Build history of the part. All positions in model axes, mm. Round coordinates to 2 decimals unless told otherwise and drop trailing zeros. Loops run counter-clockwise (first coordinate to the right, second up) from the corner with the lowest first, then second, coordinate; pieces in that order, holes last. Notation, with made-up numbers: (-27.5, -6) - (26.5, -6) arc R21 ccw to (26.5, 28) - close; hole circle Ø8 at (60.5, 83). An arc over 180 degrees is marked (long way). Use a Markdown table: item, result.
from build123d import *

# Parameters (mm, degrees)
F0_W     = 1
F0_H     = 5
F1_DEPTH = 2
F2_DEPTH = 2


# Not quite as in the source:
# - a feature names something its author has since deleted; it is built from what else it names


with BuildPart() as f1:
    # F0 (on Front) → F1 (new body)
    with BuildSketch(Plane.XZ):
        Polygon((-11.0105917081, 20.8667229116), (-10.0105917081, 20.8667229116), (-10.0105917081, 15.8667229116), (-10.0105917081, -14.7727085277), (-10.0105917081, -21.2332770884), (9.9894082919, -21.2332770884), (9.9894082919, -23.2332770884), (37.9894082919, -23.2332770884), (65.9894082919, -23.2332770884), (65.9894082919, -21.2332770884), (85.9894082919, -21.2332770884), (85.9894082919, -14.7727085277), (85.9894082919, 15.8667229116), (98.9894082919, 15.8667229116), (103.9894082919, 15.8667229116), (105.0934082919, 15.8667229116), (105.0934082919, 42.8667229116), (103.9894082919, 42.8667229116), (98.9894082919, 42.8667229116), (93.9894082919, 42.8667229116), (37.9894082919, 42.8667229116), (-10.0105917081, 42.8667229116), (-11.0105917081, 42.8667229116), align=None)
        with BuildLine():
            ThreePointArc((46.4894082919, 29.3667229116), (45.4894082919, 28.3667229116), (44.4894082919, 29.3667229116))
            ThreePointArc((44.4894082919, 29.3667229116), (45.4894082919, 30.3667229116), (46.4894082919, 29.3667229116))
        make_face(mode=Mode.SUBTRACT)
        with BuildLine():
            ThreePointArc((93.9894082919, 28.3667229116), (93.2823015107, 30.0738296928), (94.9894082919, 29.3667229116))
            ThreePointArc((94.9894082919, 29.3667229116), (94.6965150731, 28.6596161304), (93.9894082919, 28.3667229116))
        make_face(mode=Mode.SUBTRACT)
        with Locations((-10.5105917081, 18.3667229116)):
            Rectangle(F0_W, F0_H)
    extrude(amount=F1_DEPTH)

    # F0 (on Front) → F2 (join)
    with BuildSketch(Plane.XZ):
        Polygon((-11.0105917081, 20.8667229116), (-10.0105917081, 20.8667229116), (-10.0105917081, 15.8667229116), (-10.0105917081, -14.7727085277), (-10.0105917081, -21.2332770884), (9.9894082919, -21.2332770884), (9.9894082919, -23.2332770884), (37.9894082919, -23.2332770884), (65.9894082919, -23.2332770884), (65.9894082919, -21.2332770884), (85.9894082919, -21.2332770884), (85.9894082919, -14.7727085277), (85.9894082919, 15.8667229116), (98.9894082919, 15.8667229116), (103.9894082919, 15.8667229116), (105.0934082919, 15.8667229116), (105.0934082919, 42.8667229116), (103.9894082919, 42.8667229116), (98.9894082919, 42.8667229116), (93.9894082919, 42.8667229116), (37.9894082919, 42.8667229116), (-10.0105917081, 42.8667229116), (-11.0105917081, 42.8667229116), align=None)
        with BuildLine():
            ThreePointArc((46.4894082919, 29.3667229116), (45.4894082919, 28.3667229116), (44.4894082919, 29.3667229116))
            ThreePointArc((44.4894082919, 29.3667229116), (45.4894082919, 30.3667229116), (46.4894082919, 29.3667229116))
        make_face(mode=Mode.SUBTRACT)
        with BuildLine():
            ThreePointArc((93.9894082919, 28.3667229116), (93.2823015107, 30.0738296928), (94.9894082919, 29.3667229116))
            ThreePointArc((94.9894082919, 29.3667229116), (94.6965150731, 28.6596161304), (93.9894082919, 28.3667229116))
        make_face(mode=Mode.SUBTRACT)
    extrude(amount=F2_DEPTH)


solid = f1.part
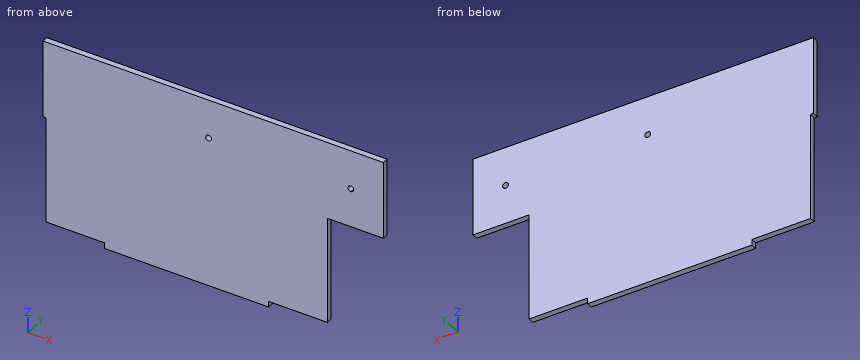
Q1. Cut at B-B, the plane z = -1. List the corners of the cut face in (x, y).
Results found:
| item | result |
|---|---|
| outline | (-10.01, -2) - (85.99, -2) - (85.99, 0) - (-10.01, 0) - close |
Q2. Drop flat-ended pins along their axis: pin 1 (0.6 mm diameter, centred on x = -1.5, y = -1, fed in from -Z); pin 2 (10 mm diameter, centred on x = 23, z = 21, fed in from +Y); pin 3 (1 mm diameter, centred on y = -0.5, z = -22.5, fed in from +X); pin 4 (1.6 mm diameter, centred on x = 45.49, z = 29.37, fed in from -Y). Give the stop position or say it passes through.
Results found:
| item | result |
|---|---|
| pin 1 | stops at z = -21.23 |
| pin 2 | stops at y = 0 |
| pin 3 | stops at x = 65.99 |
| pin 4 | passes through |
Q3. Cut at A-A, the plane y = -1.15. List the corners of the cut face in (x, z).
Results found:
| item | result |
|---|---|
| outline | (-11.01, 15.87) - (-10.01, 15.87) - (-10.01, -21.23) - (9.99, -21.23) - (9.99, -23.23) - (65.99, -23.23) - (65.99, -21.23) - (85.99, -21.23) - (85.99, 15.87) - (105.09, 15.87) - (105.09, 42.87) - (-11.01, 42.87) - close; hole circle Ø2 at (45.49, 29.37); hole circle Ø2 at (93.99, 29.37) |
Q4. Cut at C-C, the plane x = 78. List the corners of the cut face in (y, z).
Results found:
| item | result |
|---|---|
| outline | (-2, -21.23) - (0, -21.23) - (0, 42.87) - (-2, 42.87) - close |
Q5. Probe line 1 (Z direction, x = 71, y = -0.95); line 2 (X direction, y = -1.7, z = 8.5); line 3 (Z direction, x = 96, y = -0.95). List the from-to ranges inside material, lowest first.
Results found:
| item | result |
|---|---|
| line 1 | z = -21.23 to 42.87 |
| line 2 | x = -10.01 to 85.99 |
| line 3 | z = 15.87 to 42.87 |
